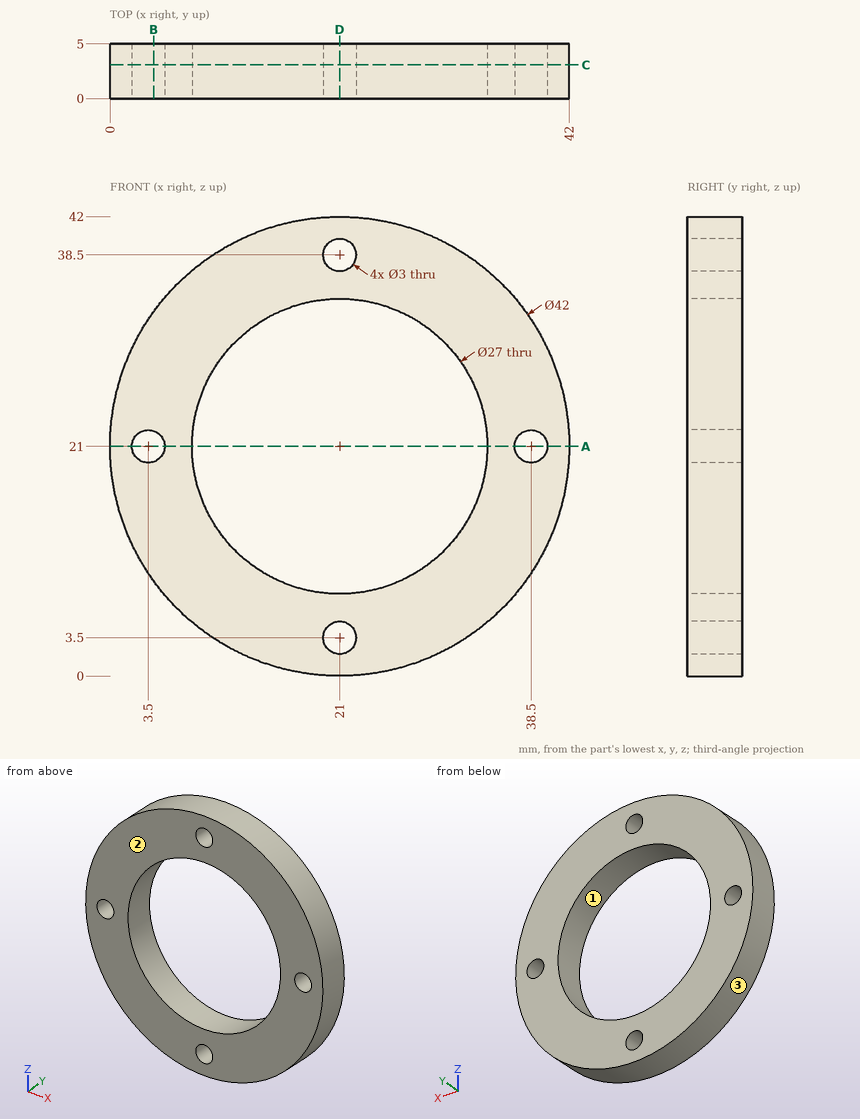
Design review of the part shown in the three views and the two pictorial views. Dimensions are in mm from the part's minimum x, y and z. Round coordinates to 2 decimals unless told otherwise and drop trailing zeros. Loops run counter-clockwise (first coordinate to the right, second up) from the corner with the lowest first, then second, coordinate; pieces in that order, holes last. Notation, with made-up numbers: (17.5, 41.25) - (66.5, 41.25) arc R18 ccw to (66.5, 48.25) - close; hole circle Ø5 at (-39, 52.25). An arc over 180 degrees is marked (long way). Use CSV: the item, a comma, the result in double quotes.
(1) Take a section at B-B, the plane x = 4. Give the boundary of the cut face in (y, z).
Working result:
outline,"(0, 8.67) - (5, 8.67) - (5, 19.59) - (0, 19.59) - close; (0, 22.41) - (5, 22.41) - (5, 33.33) - (0, 33.33) - close"
(2) The part is to be moulded in two halves that separate along X. For the marked faces 1, 2 and 3, say which applies: pulls with the +X half, pulls with the -X half, needs draft (parallel to the pull), parting line crosses it, or undercut.
Working result:
face 1,"undercut"
face 2,"needs draft"
face 3,"parting line crosses it"
(3) Take a section at C-C, the plane y = 3.1. Give the boundary of the cut face in (x, z).
Working result:
outline,"circle Ø42 at (21, 21); hole circle Ø3 at (3.5, 21); hole circle Ø27 at (21, 21); hole circle Ø3 at (21, 3.5); hole circle Ø3 at (21, 38.5); hole circle Ø3 at (38.5, 21)"
(4) Take a section at D-D, the plane x = 21. Give the boundary of the cut face in (y, z).
Working result:
outline,"(0, 0) - (5, 0) - (5, 2) - (0, 2) - close; (0, 5) - (5, 5) - (5, 7.5) - (0, 7.5) - close; (0, 34.5) - (5, 34.5) - (5, 37) - (0, 37) - close; (0, 40) - (5, 40) - (5, 42) - (0, 42) - close"
(5) For line 1 (X direction, y = 3.2, z = 21); line 2 (Z direction, x = 14.5, y = 1.2); line 3 (Z direction, x = 29, y = 4.1), list the stretches that pass through material, from the lowest coordinate up.
Working result:
line 1,"x = 0 to 2, 5 to 7.5, 34.5 to 37, 40 to 42"
line 2,"z = 1.03 to 9.17, 32.83 to 40.97"
line 3,"z = 1.58 to 10.13, 31.87 to 40.42"
(6) Take a section at A-A, the plane z = 21. Give the boundary of the cut face in (x, y), plus the area to 3 significant figures.
Working result:
outline,"(0, 0) - (2, 0) - (2, 5) - (0, 5) - close; (5, 0) - (7.5, 0) - (7.5, 5) - (5, 5) - close; (34.5, 0) - (37, 0) - (37, 5) - (34.5, 5) - close; (40, 0) - (42, 0) - (42, 5) - (40, 5) - close"
area,"45.0 mm^2"
(7) Clearance check with flat-ended pins moving along their axes: P1, Ø2.5, axis at x = 38.5, z = 21, coming from the -Y side; P2, Ø2, axis at y = 1, z = 30.5, coming from the -X side; P3, Ø1, axis at y = 2.5, z = 29.5, coming from the -X side. State where each tip first meets the part, or that it passes through.
Working result:
P1,"passes through"
P2,"stops at x = 1.8"
P3,"stops at x = 1.58"
